Can you work these out from the model? Positions are in its coordinate system, mm. Coordinates: 2 decimals unless noted, no trailing zeros. Order: outer loops, then holes, each group sorted by start corner. A loop starts at its lowest first (then second) coordinate and runs counter-clockwise, first axis right, second up. Notation, with made-up numbers: (-13, 78.25) -> (2, 78.25) arc R20 ccw to (2, 110.25) -> close; hole circle Ø3 at (66.5, 1.25). An arc over 180 degrees is marked (long way). Return JSON: item names as keys, results as strings. Group by question number.
1) For pin 1 (3.5 mm diameter, centred on x = 70, z = -3.32, fed in from -Y), with a flat end and sliding along its axis, tell me the tip position at first contact or that it passes through.
2) If we section it at B-B, the plane y = 0.6: State how many separate pieces and enclosed holes the cut face has, then the cut area to 3 significant figures.
3) If I drill on probe 1 along Z at (x, y) = (250, 1.25); probe 2 along X at (y, z) = (1.7, -23.5); probe 3 along X at (y, z) = (1.4, -99), over which ranges is the centre line in solid material (lowest first)? Write a range as from..to.
4) If we section it at A-A, the plane x = 121: Please give me the cut outline in (y, z).
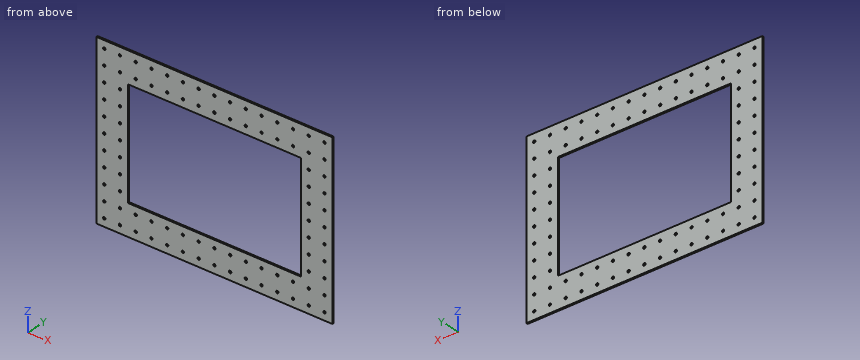
from build123d import *

# Parameters (mm, degrees)
SKETCH1_W           = 220
SKETCH1_H           = 2
BOSS_EXTRUDE1_DEPTH = 300
SKETCH2_R           = 1.5
SKETCH2_W           = 220
SKETCH2_H           = 140
CUT_EXTRUDE1_DEPTH  = 10


with BuildPart() as part:
    # Sketch1 → Boss-Extrude1 (new body)
    with BuildSketch(Plane(origin=(0, 0, 0), x_dir=(0, 0, -1), z_dir=(1, 0, 0))):
        with Locations((83.3216851, 1)):
            Rectangle(SKETCH1_W, SKETCH1_H)
    extrude(amount=BOSS_EXTRUDE1_DEPTH)

    # Sketch2 → Cut-Extrude1 (cut)
    with BuildSketch(Plane(origin=(0, 2, 0), x_dir=(1, 0, 0), z_dir=(0, 1, 0))):
        with Locations((10, -16.6783149)):
            Circle(SKETCH2_R)
        with Locations((30, -16.6783149)):
            Circle(SKETCH2_R)
        with Locations((50, -16.6783149)):
            Circle(SKETCH2_R)
        with Locations((70, -16.6783149)):
            Circle(SKETCH2_R)
        with Locations((90, -16.6783149)):
            Circle(SKETCH2_R)
        with Locations((110, -16.6783149)):
            Circle(SKETCH2_R)
        with Locations((130, -16.6783149)):
            Circle(SKETCH2_R)
        with Locations((150, -16.6783149)):
            Circle(SKETCH2_R)
        with Locations((170, -16.6783149)):
            Circle(SKETCH2_R)
        with Locations((190, -16.6783149)):
            Circle(SKETCH2_R)
        with Locations((210, -16.6783149)):
            Circle(SKETCH2_R)
        with Locations((230, -16.6783149)):
            Circle(SKETCH2_R)
        with Locations((250, -16.6783149)):
            Circle(SKETCH2_R)
        with Locations((270, -16.6783149)):
            Circle(SKETCH2_R)
        with Locations((290, -16.6783149)):
            Circle(SKETCH2_R)
        with Locations((10, 3.3216851)):
            Circle(SKETCH2_R)
        with Locations((270, 3.3216851)):
            Circle(SKETCH2_R)
        with Locations((290, 3.3216851)):
            Circle(SKETCH2_R)
        with Locations((10, 23.3216851)):
            Circle(SKETCH2_R)
        with Locations((30, 23.3216851)):
            Circle(SKETCH2_R)
        with Locations((270, 23.3216851)):
            Circle(SKETCH2_R)
        with Locations((290, 23.3216851)):
            Circle(SKETCH2_R)
        with Locations((10, 43.3216851)):
            Circle(SKETCH2_R)
        with Locations((30, 43.3216851)):
            Circle(SKETCH2_R)
        with Locations((270, 43.3216851)):
            Circle(SKETCH2_R)
        with Locations((290, 43.3216851)):
            Circle(SKETCH2_R)
        with Locations((10, 63.3216851)):
            Circle(SKETCH2_R)
        with Locations((30, 63.3216851)):
            Circle(SKETCH2_R)
        with Locations((270, 63.3216851)):
            Circle(SKETCH2_R)
        with Locations((290, 63.3216851)):
            Circle(SKETCH2_R)
        with Locations((10, 83.3216851)):
            Circle(SKETCH2_R)
        with Locations((30, 83.3216851)):
            Circle(SKETCH2_R)
        with Locations((270, 83.3216851)):
            Circle(SKETCH2_R)
        with Locations((290, 83.3216851)):
            Circle(SKETCH2_R)
        with Locations((10, 103.3216851)):
            Circle(SKETCH2_R)
        with Locations((30, 103.3216851)):
            Circle(SKETCH2_R)
        with Locations((270, 103.3216851)):
            Circle(SKETCH2_R)
        with Locations((290, 103.3216851)):
            Circle(SKETCH2_R)
        with Locations((10, 123.3216851)):
            Circle(SKETCH2_R)
        with Locations((30, 123.3216851)):
            Circle(SKETCH2_R)
        with Locations((270, 123.3216851)):
            Circle(SKETCH2_R)
        with Locations((290, 123.3216851)):
            Circle(SKETCH2_R)
        with Locations((10, 143.3216851)):
            Circle(SKETCH2_R)
        with Locations((30, 143.3216851)):
            Circle(SKETCH2_R)
        with Locations((270, 143.3216851)):
            Circle(SKETCH2_R)
        with Locations((290, 143.3216851)):
            Circle(SKETCH2_R)
        with Locations((10, 163.3216851)):
            Circle(SKETCH2_R)
        with Locations((30, 163.3216851)):
            Circle(SKETCH2_R)
        with Locations((290, 163.3216851)):
            Circle(SKETCH2_R)
        with Locations((10, 183.3216851)):
            Circle(SKETCH2_R)
        with Locations((30, 183.3216851)):
            Circle(SKETCH2_R)
        with Locations((50, 183.3216851)):
            Circle(SKETCH2_R)
        with Locations((70, 183.3216851)):
            Circle(SKETCH2_R)
        with Locations((90, 183.3216851)):
            Circle(SKETCH2_R)
        with Locations((110, 183.3216851)):
            Circle(SKETCH2_R)
        with Locations((130, 183.3216851)):
            Circle(SKETCH2_R)
        with Locations((150, 183.3216851)):
            Circle(SKETCH2_R)
        with Locations((170, 183.3216851)):
            Circle(SKETCH2_R)
        with Locations((190, 183.3216851)):
            Circle(SKETCH2_R)
        with Locations((210, 183.3216851)):
            Circle(SKETCH2_R)
        with Locations((230, 183.3216851)):
            Circle(SKETCH2_R)
        with Locations((250, 183.3216851)):
            Circle(SKETCH2_R)
        with Locations((270, 183.3216851)):
            Circle(SKETCH2_R)
        with Locations((290, 183.3216851)):
            Circle(SKETCH2_R)
        with Locations((50, 163.3216851)):
            Circle(SKETCH2_R)
        with Locations((70, 163.3216851)):
            Circle(SKETCH2_R)
        with Locations((90, 163.3216851)):
            Circle(SKETCH2_R)
        with Locations((110, 163.3216851)):
            Circle(SKETCH2_R)
        with Locations((130, 163.3216851)):
            Circle(SKETCH2_R)
        with Locations((150, 163.3216851)):
            Circle(SKETCH2_R)
        with Locations((170, 163.3216851)):
            Circle(SKETCH2_R)
        with Locations((190, 163.3216851)):
            Circle(SKETCH2_R)
        with Locations((210, 163.3216851)):
            Circle(SKETCH2_R)
        with Locations((230, 163.3216851)):
            Circle(SKETCH2_R)
        with Locations((250, 163.3216851)):
            Circle(SKETCH2_R)
        with Locations((30, 3.3216851)):
            Circle(SKETCH2_R)
        with Locations((50, 3.3216851)):
            Circle(SKETCH2_R)
        with Locations((70, 3.3216851)):
            Circle(SKETCH2_R)
        with Locations((90, 3.3216851)):
            Circle(SKETCH2_R)
        with Locations((110, 3.3216851)):
            Circle(SKETCH2_R)
        with Locations((130, 3.3216851)):
            Circle(SKETCH2_R)
        with Locations((150, 3.3216851)):
            Circle(SKETCH2_R)
        with Locations((170, 3.3216851)):
            Circle(SKETCH2_R)
        with Locations((190, 3.3216851)):
            Circle(SKETCH2_R)
        with Locations((210, 3.3216851)):
            Circle(SKETCH2_R)
        with Locations((230, 3.3216851)):
            Circle(SKETCH2_R)
        with Locations((250, 3.3216851)):
            Circle(SKETCH2_R)
        with Locations((270, 163.3216851)):
            Circle(SKETCH2_R)
        with Locations((150, 83.3216851)):
            Rectangle(SKETCH2_W, SKETCH2_H)
    extrude(amount=-CUT_EXTRUDE1_DEPTH, mode=Mode.SUBTRACT)


solid = part.part
Result sheet:
{
 "1": {"pin 1": "stops at y = 0"},
 "2": {"separate pieces": "1", "enclosed holes": "89", "area": "34,600 mm2"},
 "3": {"probe 1": "z = -193.32..-184.82, -181.82..-164.82, -161.82..-153.32, -13.32..-4.82, -1.82..15.18, 18.18..26.68", "probe 2": "x = 0..8.51, 11.49..28.51, 31.49..40, 260..268.51, 271.49..288.51, 291.49..300", "probe 3": "x = 0..40, 260..300"},
 "4": {"outline": "(0, -193.32) -> (2, -193.32) -> (2, -153.32) -> (0, -153.32) -> close; (0, -13.32) -> (2, -13.32) -> (2, 26.68) -> (0, 26.68) -> close"}
}
